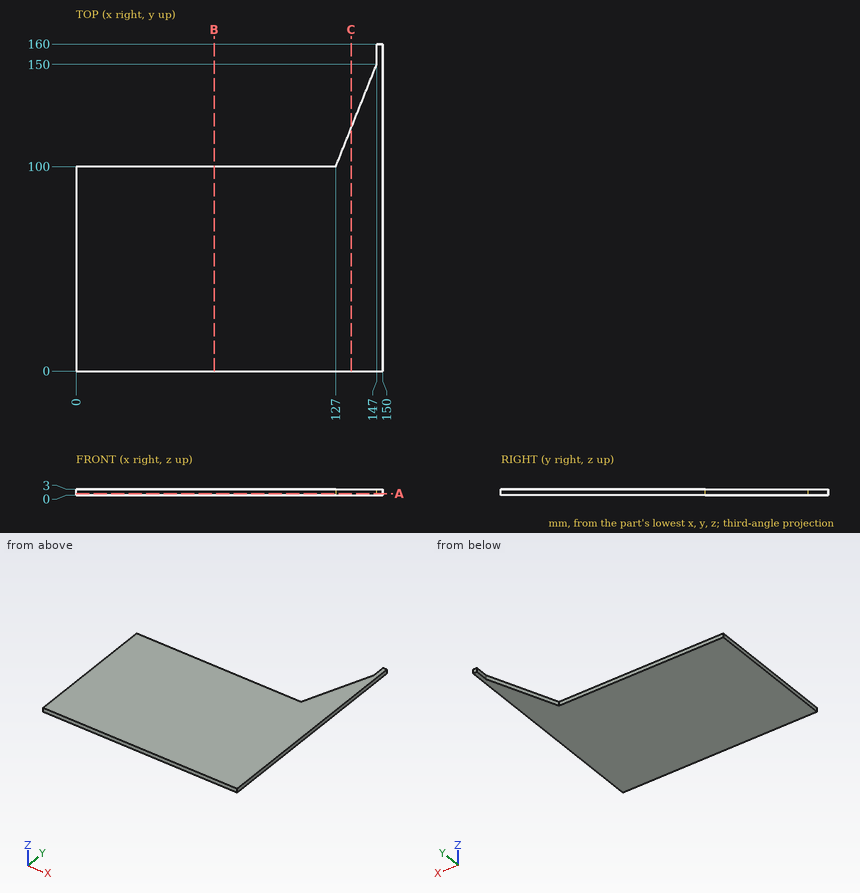
Can you work these out from the drawing? Everything is in mm from the part's minimum corner. Round coordinates to 2 decimals unless told otherwise and drop trailing zeros. Loops run counter-clockwise (first coordinate to the right, second up) from the corner with the lowest first, then second, coordinate; pieces in that order, holes last. Notation, with made-up numbers: (64.5, 78) -> (107.5, 78) arc R11 ccw to (107.5, 98) -> close; hole circle Ø4 at (10, 46). An arc over 180 degrees is marked (long way). Use CSV: the item, a comma, the result in double quotes.
(1) Will this pin go through, and if not, where does the flat tip stop? pin 1 Ø1.5 at (x, z) = (91, 1) entering from +Y.
Return value:
pin 1,"stops at y = 100"
(2) If I drill on probe 1 along Y at (x, z) = (19, 0.65); probe 2 along X at (y, z) = (111.5, 1.8); probe 3 along X at (y, z) = (102, 0.65), over which ranges is the centre line in solid material (lowest first)? Write a range as [from, to].
Return value:
probe 1,"y = [0, 100]"
probe 2,"x = [131.6, 150]"
probe 3,"x = [127.8, 150]"
(3) Suppose I cut it at C-C on x = 134.5. Write out the boundary of the cut face in (y, z).
Return value:
outline,"(0, 0) -> (118.75, 0) -> (118.75, 3) -> (0, 3) -> close"
(4) Suppose I cut it at B-B on x = 67.5. Write out the boundary of the cut face in (y, z), plus the area to 3 significant figures.
Return value:
outline,"(0, 0) -> (100, 0) -> (100, 3) -> (0, 3) -> close"
area,"300 mm²"
(5) Suppose I cut it at A-A on z = 0.85. Write out the boundary of the cut face in (x, y), plus the area to 3 significant figures.
Return value:
outline,"(0, 0) -> (150, 0) -> (150, 160) -> (147, 160) -> (147, 150) -> (127, 100) -> (0, 100) -> close"
area,"15,700 mm²"
